Autodesk Inventor part; units mm, degrees
ref_plane "YZ Plane" through (0, 0, 0) normal (1, 0, 0) x (0, 1, 0)
ref_plane "XZ Plane" through (0, 0, 0) normal (0, 1, 0) x (-1, 0, 0)
ref_plane "XY Plane" through (0, 0, 0) normal (0, 0, 1) x (1, 0, 0)
sketch "Sketch1" plane through (0, 0, 0) normal (0, 0, 1) x (1, 0, 0)
  circle A0 centre (0, 0) radius 4.51
  line L0 (-0.0588, 9.8148) -> (8.4705, 4.9583)
  line L1 (8.4705, 4.9583) -> (8.5292, -4.8565)
  line L2 (8.5292, -4.8565) -> (0.0588, -9.8148)
  line L3 (0.0588, -9.8148) -> (-8.4705, -4.9583)
  line L4 (-8.4705, -4.9583) -> (-8.5292, 4.8565)
  line L5 (-8.5292, 4.8565) -> (-0.0588, 9.8148)
  dimension "d0" = 9.02
  dimension "d1" = 8.5
extrude "Extrusion1" add sketch "Sketch1" along normal blind 5
chamfer "Chamfer1" distance 0.6 angle 45 14 edges at (-4.294, 7.3356, 5) (-8.4998, -0.0509, 5) (-4.2058, -7.3865, 5) (4.294, -7.3356, 5) (8.4998, 0.0509, 5) (4.2058, 7.3865, 5) (-4.2058, -7.3865, 0) (4.294, -7.3356, 0) (8.4998, 0.0509, 0) (4.2058, 7.3865, 0) (-4.294, 7.3356, 0) (-8.4998, -0.0509, 0) (-4.51, 0, 5) (-4.51, 0, 0)
properties part number "TuercaManzana" material "Steel"
Here's how the part is built. I have some questions about the finished solid (model axes, mm). Round coordinates to 2 decimals unless told otherwise and drop trailing zeros. Order: outer loops, then holes, each group sorted by start corner. A loop starts at its lowest first (then second) coordinate and runs counter-clockwise, first axis right, second up. Notation, with made-up numbers: (87, -23.5) -> (125, -23.5) arc R33 ccw to (125, 8.5) -> close; hole circle Ø2 at (87, 9). An arc over 180 degrees is marked (long way). Use CSV: the item, a comma, the result in double quotes.
1. I want a section at B-B on y = 0. List the corners of the cut face in (x, z) for me.
Recorded:
outline,"(-8.5, 0.6) -> (-7.9, 0) -> (-5.11, 0) -> (-4.51, 0.6) -> (-4.51, 4.4) -> (-5.11, 5) -> (-7.9, 5) -> (-8.5, 4.4) -> close; (4.51, 0.6) -> (5.11, 0) -> (7.9, 0) -> (8.5, 0.6) -> (8.5, 4.4) -> (7.9, 5) -> (5.11, 5) -> (4.51, 4.4) -> close"
2. Thinking about a two-plate mould opening in X: for faces 1 (the face through (-4, -4, 0)), 2 (the face through (4.15, 7.42, 2.47)), 3 (the face through (-4.15, -7.42, 2.47)), 4 (the face through (4.166, 1.727, 2.473)), which applies, pulls with the +X half, pulls with the -X half, needs draft (parallel to the pull), parting line crosses it, or undercut?
Recorded:
face 1,"needs draft"
face 2,"pulls with the +X half"
face 3,"pulls with the -X half"
face 4,"undercut"
3. I want a section at A-A on z = 2.6. List the corners of the cut face in (x, y) for me, and give its area (3 significant figures).
Recorded:
outline,"(-8.53, 4.86) -> (-8.47, -4.96) -> (0.06, -9.81) -> (8.53, -4.86) -> (8.47, 4.96) -> (-0.06, 9.81) -> close; hole circle Ø9.02 at (0, 0)"
area,"186 mm2"
4. I need wall thicknesses on line 1 along Y through (x, z) = (-4, 2.4); line 2 along X through (y, z) = (2.25, 0.5); line 3 along Y through (x, z) = (-3.25, 2.5). Which ranges of each line are inside material? Lowest first, please.
Recorded:
line 1,"y = -7.5 to -2.08, 2.08 to 7.51"
line 2,"x = -8.41 to -4.02, 4.02 to 8.39"
line 3,"y = -7.93 to -3.13, 3.13 to 7.95"
5. I'm going to push flat-ended pins straight in: P1, Ø1.5, axis at y = 6, z = 4, coming from the +X side; P2, Ø3, axis at x = -6, z = 2.5, coming from the +Y side; P3, Ø1.5, axis at x = 3.5, z = 1, coming from the +Y side. Where does each tip first touch, or does it pass through?
Recorded:
P1,"stops at x = 7.96"
P2,"stops at y = 7.22"
P3,"stops at y = 8.22"
